Verification items for the finished model (mm, model axes). A direction names the side the tool comes from. Give positions to 0.01 mm unless a question says otherwise; leave off trailing zeros.
(1) Access from +Z, -Z, +X, -X, +Y, -Y to the whole of each face (thin tool, end or side, straight path). Record for faces 4 (the face through (-10.122, 3.072, -0.986)), 5 (the face through (-14.4, 5.21, -2.96)).
(2) Gauge pin test, flat ends, axial feed: pin 1 (1.5 mm diameter, centred on y = 13, z = -5, fed in from +X) (3 decimals); pin 2 (1.5 mm diameter, centred on y = 6, z = -3, fed in from +X); pin 3 (3 mm diameter, centred on x = 6, z = -2.5, fed in from -Y). Record the tip position at first contact, or that the pin passes through.
(3) Scan lines: L1, parallel to Y at x = 0, z = -5.15; L2, parallel to Y at x = 17, z = -4; L3, parallel to X at y = 12.5, z = -2.25. Record each from-to range of solid material in increasing order.
(4) Mould release check, pull along Y, two halves, no side actions. Record for faces 1 (the face through (19.84, -15.68, -2.96)), 2 (the face through (-29.97, 1.32, -0.63)), 3 (the face through (-7.1, 0.4, -6)): pulls with the +Y half, pulls with the -Y half, needs draft (parallel to the pull), parting line crosses it, or undercut.
(5) Sectioned sample at A-A on y = -11. Count the separate pieces of the cut face and the enclosed holes in it, plus the area to 3 significant figures.
```python
from build123d import *

# Parameters (mm, degrees)
SKETCH1_R           = 30
SKETCH1_R_2         = 7.7
SKETCH1_R_3         = 2.3
SKETCH1_R_4         = 0.6
BOSS_EXTRUDE1_DEPTH = 6
CUT_EXTRUDE1_DEPTH  = 2


with BuildPart() as part:
    # Sketch1 → Boss-Extrude1 (new body)
    with BuildSketch(Plane.XY):
        Circle(SKETCH1_R)
        with Locations((-12.727922061, 12.727922061)):
            Circle(SKETCH1_R_2, mode=Mode.SUBTRACT)
        with Locations((12.727922061, 12.727922061)):
            Circle(SKETCH1_R_2, mode=Mode.SUBTRACT)
        with Locations((12.727922061, -12.727922061)):
            Circle(SKETCH1_R_2, mode=Mode.SUBTRACT)
        with Locations((-12.727922061, -12.727922061)):
            Circle(SKETCH1_R_2, mode=Mode.SUBTRACT)
        Circle(SKETCH1_R_3, mode=Mode.SUBTRACT)
        with Locations((-14.85, 0)):
            Circle(SKETCH1_R_4, mode=Mode.SUBTRACT)
        with Locations((6.45, 0)):
            Circle(SKETCH1_R_4, mode=Mode.SUBTRACT)
        with Locations((0, -6.45)):
            Circle(SKETCH1_R_4, mode=Mode.SUBTRACT)
        with Locations((-6.45, 0)):
            Circle(SKETCH1_R_4, mode=Mode.SUBTRACT)
        with Locations((0, 6.45)):
            Circle(SKETCH1_R_4, mode=Mode.SUBTRACT)
        with Locations((0, 14.85)):
            Circle(SKETCH1_R_4, mode=Mode.SUBTRACT)
        with Locations((14.85, 0)):
            Circle(SKETCH1_R_4, mode=Mode.SUBTRACT)
        with Locations((0, -14.85)):
            Circle(SKETCH1_R_4, mode=Mode.SUBTRACT)
    extrude(amount=-BOSS_EXTRUDE1_DEPTH)

    # Cut-Sweep1: sweep along a curve in space
    with BuildLine() as cut_sweep1_path:
        ThreePointArc((30, 0, -6), (21.213203436, 21.213203436, -6), (0, 30, -6))
        ThreePointArc((0, 30, -6), (-21.213203436, 21.213203436, -6), (-30, 0, -6))
        ThreePointArc((-30, 0, -6), (-21.213203436, -21.213203436, -6), (0, -30, -6))
        ThreePointArc((0, -30, -6), (21.213203436, -21.213203436, -6), (30, 0, -6))
    # Sketch2 → Cut-Sweep1 (sweep, cut)
    with BuildSketch(Plane(origin=(0, 0, 0), x_dir=(1, 0, 0), z_dir=(0, 1, 0))):
        Polygon((-31.156921938, 0.6), (-27, 3), (-31.156921938, 5.4), align=None)
    sweep(path=cut_sweep1_path.line, mode=Mode.SUBTRACT)

    # Sketch4 → Cut-Extrude1 (cut)
    with BuildSketch(Plane.XY):
        with BuildLine():
            Line((-3.770723751, 3.831893278), (-16.652735562, 2.291047422))
            ThreePointArc((-16.652735562, 2.291047422), (-18.75, 0), (-16.652735562, -2.291047422))
            Line((-16.652735562, -2.291047422), (-3.831893278, -3.770723751))
            Line((-3.831893278, -3.770723751), (-2.291047422, -16.652735562))
            ThreePointArc((-2.291047422, -16.652735562), (0, -18.75), (2.291047422, -16.652735562))
            Line((2.291047422, -16.652735562), (3.770723751, -3.831893278))
            Line((3.770723751, -3.831893278), (16.652735562, -2.291047422))
            ThreePointArc((16.652735562, -2.291047422), (18.75, 0), (16.652735562, 2.291047422))
            Line((16.652735562, 2.291047422), (3.831893278, 3.770723751))
            Line((3.831893278, 3.770723751), (2.291047422, 16.652735562))
            ThreePointArc((2.291047422, 16.652735562), (0, 18.75), (-2.291047422, 16.652735562))
            Line((-2.291047422, 16.652735562), (-3.770723751, 3.831893278))
        make_face()
    extrude(amount=-CUT_EXTRUDE1_DEPTH, mode=Mode.SUBTRACT)


solid = part.part
```
Ans:
1. face 4: +Z
1. face 5: +Z, -Z
2. pin 1: stops at x = 27.385
2. pin 2: stops at x = 27.67
2. pin 3: stops at y = -29.56
3. L1: y = -30 to -15.45, -14.25 to -7.05, -5.85 to -2.3, 2.3 to 5.85, 7.05 to 14.25, 15.45 to 30
3. L2: y = -23.16 to -19.13, -6.32 to 6.32, 19.13 to 23.16
3. L3: x = -25.39 to -20.42, -5.03 to 5.03, 20.42 to 25.39
4. face 1: undercut
4. face 2: parting line crosses it
4. face 3: needs draft
5. separate pieces: 3
5. enclosed holes: 0
5. area: 132 mm2
